Can you work these out from the drawing? Everything is in mm from the part's minimum corner. Round coordinates to 2 decimals unless told otherwise and drop trailing zeros. Order: outer loops, then holes, each group sorted by start corner. A loop starts at its lowest first (then second) coordinate and runs counter-clockwise, first axis right, second up. Notation, with made-up numbers: (1.5, 12) - (36.5, 12) arc R17 cw to (36.5, 35) - close; hole circle Ø8 at (-24, 36). An arc over 180 degrees is marked (long way). Answer as a JSON object with one key per item and string values.
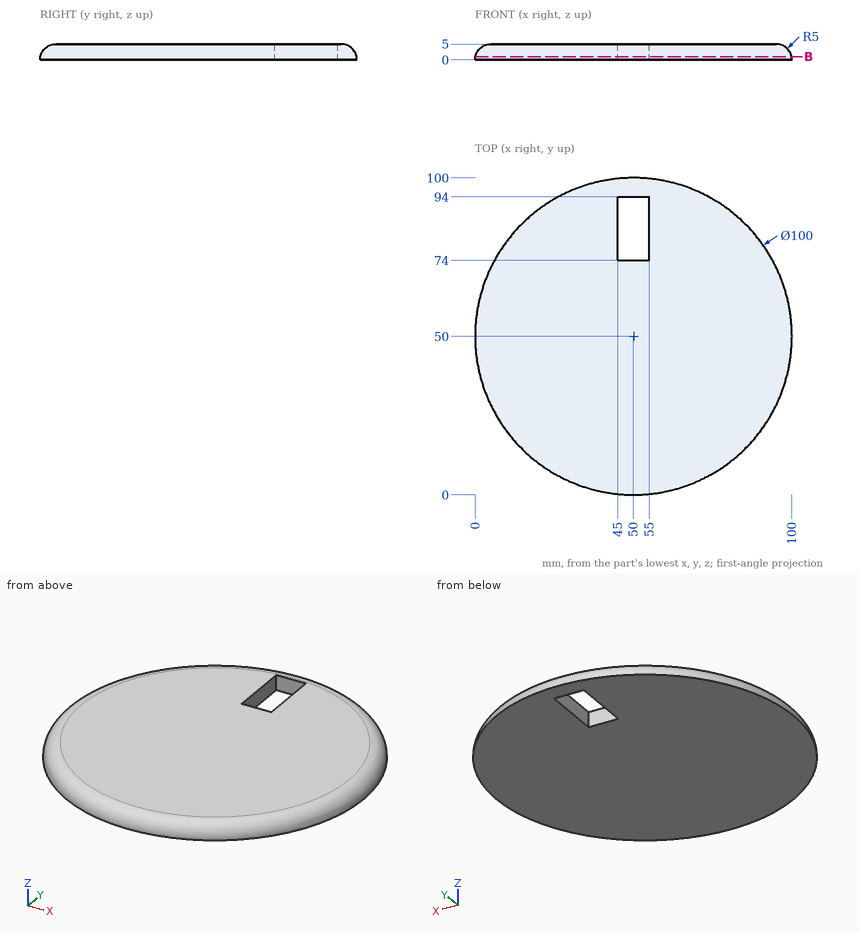
1. If I drill on L1, parallel to X at y = 83.5, z = 4.1; L2, parallel to X at y = 86.5, z = 1.5; L3, parallel to Y at x = 50, z = 1.75, over which ranges is the centre line in solid material (lowest first)? Write a range as [from, to].
Responses:
{"L1": "[15.82, 45], [55, 84.18]", "L2": "[16.17, 45], [55, 83.83]", "L3": "[0.32, 74], [94, 99.68]"}
2. For P1, Ø8, axis at x = 53, y = 55, coming from the -Z side; P2, Ø1, axis at x = 11, z = 3, coming from the -Y side; P3, Ø2.5, axis at x = 49.5, z = 2, coming from the -Y side; P4, Ø1.5, axis at x = 48.5, z = 2.5, coming from the +Y side, each with a flat end and sliding along its axis, tell me the tip position at first contact or that it passes through.
Responses:
{"P1": "z = 0", "P2": "y = 19.48", "P3": "y = 0.06", "P4": "y = 99.66"}
3. Imagine slicing it at B-B (z = 1). List the corners of the cut face in (x, y) for me, plus the area to 3 significant figures.
Responses:
{"outline": "circle Ø99.8 at (50, 50); hole (45, 74) - (55, 74) - (55, 94) - (45, 94) - close", "area": "7,620 mm2"}
